Geometry check sheet. Reference: the model listing, model coordinates, mm. Face numbers are marked on the shaded views. A direction names the side the tool comes from. Coordinates: 2 decimals unless noted, no trailing zeros. Order: outer loops, then holes, each group sorted by start corner. A loop starts at its lowest first (then second) coordinate and runs counter-clockwise, first axis right, second up.
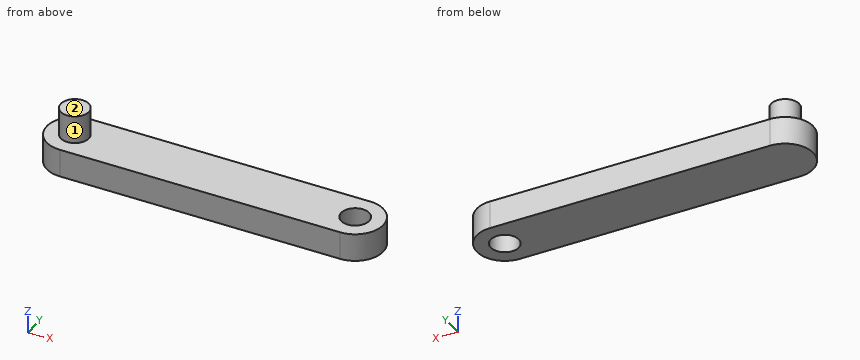
```python
from build123d import *

# Parameters (mm, degrees)
SKETCH1_R           = 2.5
BOSS_EXTRUDE1_DEPTH = 5
SKETCH1_2_R         = 2.5
BOSS_EXTRUDE2_DEPTH = 10


with BuildPart() as part:
    # Sketch1 → Boss-Extrude1 (new body)
    with BuildSketch(Plane.XY):
        with BuildLine():
            Line((-25, 5), (25, 5))
            ThreePointArc((25, 5), (30, 0), (25, -5))
            Line((25, -5), (-25, -5))
            ThreePointArc((-25, -5), (-30, 0), (-25, 5))
        make_face()
        with Locations((-25, 0)):
            Circle(SKETCH1_R, mode=Mode.SUBTRACT)
        with Locations((25, 0)):
            Circle(SKETCH1_R, mode=Mode.SUBTRACT)
    extrude(amount=BOSS_EXTRUDE1_DEPTH)

    # Sketch1<2> → Boss-Extrude2 (add)
    with BuildSketch(Plane.XY):
        with Locations((-25, 0)):
            Circle(SKETCH1_2_R)
    extrude(amount=BOSS_EXTRUDE2_DEPTH)


solid = part.part
```
Item 1: Sectioned sample at D-D (z = 8.5). Record the cut outline in (x, y), and give its area (3 significant figures).
Item 2: Thickness scan on line 1 along Y through (x, z) = (25, 3.15); line 2 along Z through (x, y) = (-12.5, -0.5); line 3 along X through (y, z) = (1, 2.5). Record the ranges inside material, lowest first.
Item 3: Depth check by flat-ended pin: P1, Ø1, axis at y = -1.5, z = 7.5, coming from the -X side; P2, Ø1.5, axis at y = -3.5, z = 5, coming from the -X side; P3, Ø5, axis at x = 2.5, y = 0.5, coming from the +Z side. Enter the tip coordinate at first touch or a pass-through.
Item 4: Sectioned sample at C-C (x = 24.5). Record the cut outline in (y, z).
Item 5: Sectioned sample at A-A (y = 0). Record the cut outline in (x, z).
Item 6: Tool access check on the marked faces 1 and 2. Record the directions out of +Z, -Z, +X, -X, +Y, -Y that give a thin tool (end or side, any length) a straight path to the whole face; none if there is none.
Item 7: Sectioned sample at B-B (z = 3.5). Record the cut outline in (x, y), and give its area (3 significant figures).
Geometry check:
1. outline: circle Ø5 at (-25, 0)
1. area: 19.6 mm2
2. line 1: y = -5 to -2.5, 2.5 to 5
2. line 2: z = 0 to 5
2. line 3: x = -29.9 to 22.71, 27.29 to 29.9
3. P1: stops at x = -27.29
3. P2: stops at x = -29.18
3. P3: stops at z = 5
4. outline: (-5, 0) - (-2.45, 0) - (-2.45, 5) - (-5, 5) - close; (2.45, 0) - (5, 0) - (5, 5) - (2.45, 5) - close
5. outline: (-30, 0) - (22.5, 0) - (22.5, 5) - (-22.5, 5) - (-22.5, 10) - (-27.5, 10) - (-27.5, 5) - (-30, 5) - close; (27.5, 0) - (30, 0) - (30, 5) - (27.5, 5) - close
6. face 1: +Z
6. face 2: +Z, +X, -X, +Y, -Y
7. outline: (-25, -5) - (25, -5) arc R5 ccw to (25, 5) - (-25, 5) arc R5 ccw to start; hole circle Ø5 at (25, 0)
7. area: 559 mm2
